from build123d import *

# Parameters (mm, degrees)
BOSS_EXTRUDE1_DEPTH = 19
BOSS_EXTRUDE2_DEPTH = 1
BOSS_EXTRUDE3_DEPTH = 1
SKETCH4_W           = 11
SKETCH4_H           = 15.2
SKETCH4_W_2         = 9
SKETCH4_H_2         = 13.2
BOSS_EXTRUDE4_DEPTH = 5
SKETCH5_W           = 9
SKETCH5_H           = 13.2
CUT_EXTRUDE1_DEPTH  = 13


with BuildPart() as part:
    # Sketch1 → Boss-Extrude1 (new body)
    with BuildSketch(Plane(origin=(0, 0, 0), x_dir=(1, 0, 0), z_dir=(0, 1, 0))):
        with BuildLine():
            Line((-13.001443325, 4.911000499), (-13.001443325, -7.088999501))
            Line((-13.001443325, -7.088999501), (-3.408667462, -11.966682937))
            Line((-3.408667462, -11.966682937), (-5.189854063, -11.966682937))
            Line((-5.189854063, -11.966682937), (-14.067067881, -7.452844668))
            Line((-14.067067881, -7.452844668), (-14.067067881, 3.911000499))
            Line((-14.067067881, 3.911000499), (-28.001443325, 3.911000499))
            Line((-28.001443325, 3.911000499), (-28.001443325, -7.452844668))
            ThreePointArc((-28.001443325, -7.452844668), (-26.679370706, -10.644610317), (-23.487605056, -11.966682937))
            Line((-23.487605056, -11.966682937), (-11.742872705, -11.966682937))
            Line((-11.742872705, -11.966682937), (-11.742872705, -12.966682937))
            Line((-11.742872705, -12.966682937), (-23.494591297, -12.966682937))
            ThreePointArc((-23.494591297, -12.966682937), (-27.388523709, -11.353763321), (-29.001443325, -7.459830909))
            Line((-29.001443325, -7.459830909), (-29.001443325, 4.911000499))
            Line((-29.001443325, 4.911000499), (-13.001443325, 4.911000499))
        make_face()
    extrude(amount=BOSS_EXTRUDE1_DEPTH)

    # Sketch2 → Boss-Extrude2 (add)
    with BuildSketch(Plane(origin=(0, 19, 0), x_dir=(1, 0, 0), z_dir=(0, 1, 0))):
        with BuildLine():
            Line((-29.001443325, 4.911000499), (-13.001443325, 4.911000499))
            Line((-13.001443325, 4.911000499), (-13.001443325, -7.088999501))
            Line((-13.001443325, -7.088999501), (-3.408667462, -11.966682937))
            Line((-3.408667462, -11.966682937), (-5.189854063, -11.966682937))
            Line((-5.189854063, -11.966682937), (-11.742872705, -12.966682937))
            Line((-11.742872705, -12.966682937), (-23.494591297, -12.966682937))
            ThreePointArc((-23.494591297, -12.966682937), (-27.388523709, -11.353763321), (-29.001443325, -7.459830909))
            Line((-29.001443325, -7.459830909), (-29.001443325, 4.911000499))
        make_face()
    extrude(amount=-BOSS_EXTRUDE2_DEPTH)

    # Sketch3 → Boss-Extrude3 (add)
    with BuildSketch(Plane(origin=(0, 0, 0), x_dir=(-1, 0, 0), z_dir=(0, -1, 0))):
        with BuildLine():
            Line((29.001443325, -7.459830909), (29.001443325, 4.911000499))
            Line((29.001443325, 4.911000499), (13.001443325, 4.911000499))
            Line((13.001443325, 4.911000499), (13.001443325, -7.088999501))
            Line((13.001443325, -7.088999501), (3.408667462, -11.966682937))
            Line((3.408667462, -11.966682937), (5.189854063, -11.966682937))
            Line((5.189854063, -11.966682937), (14.067067881, -7.452844668))
            Line((14.067067881, -7.452844668), (14.067067881, 3.911000499))
            Line((14.067067881, 3.911000499), (28.001443325, 3.911000499))
            Line((28.001443325, 3.911000499), (28.001443325, -7.452844668))
            ThreePointArc((28.001443325, -7.452844668), (26.679370706, -10.644610317), (23.487605056, -11.966682937))
            Line((23.487605056, -11.966682937), (11.742872705, -11.966682937))
            Line((11.742872705, -11.966682937), (11.742872705, -12.966682937))
            Line((11.742872705, -12.966682937), (23.494591297, -12.966682937))
            ThreePointArc((23.494591297, -12.966682937), (27.388523709, -11.353763321), (29.001443325, -7.459830909))
        make_face()
        with BuildLine():
            Line((11.742872705, -12.966682937), (3.408667462, -11.966682937))
            Line((3.408667462, -11.966682937), (5.189854063, -11.966682937))
            Line((5.189854063, -11.966682937), (14.067067881, -7.452844668))
            Line((14.067067881, -7.452844668), (14.067067881, 3.911000499))
            Line((14.067067881, 3.911000499), (28.001443325, 3.911000499))
            Line((28.001443325, 3.911000499), (28.001443325, -7.452844668))
            ThreePointArc((28.001443325, -7.452844668), (26.679370706, -10.644610317), (23.487605056, -11.966682937))
            Line((23.487605056, -11.966682937), (11.742872705, -11.966682937))
            Line((11.742872705, -11.966682937), (11.742872705, -12.966682937))
        make_face()
    extrude(amount=-BOSS_EXTRUDE3_DEPTH)

    # Sketch4 → Boss-Extrude4 (add)
    with BuildSketch(Plane(origin=(0, 0, -4.911000499), x_dir=(-1, 0, 0), z_dir=(0, 0, -1))):
        with Locations((21.001443325, 9.5)):
            Rectangle(SKETCH4_W, SKETCH4_H)
        with Locations((21.001443325, 9.5)):
            Rectangle(SKETCH4_W_2, SKETCH4_H_2, mode=Mode.SUBTRACT)
    extrude(amount=BOSS_EXTRUDE4_DEPTH)

    # Sketch5 → Cut-Extrude1 (cut)
    with BuildSketch(Plane(origin=(0, 0, -9.911000499), x_dir=(-1, 0, 0), z_dir=(0, 0, -1))):
        with Locations((21.001443325, 9.5)):
            Rectangle(SKETCH5_W, SKETCH5_H)
    extrude(amount=-CUT_EXTRUDE1_DEPTH, mode=Mode.SUBTRACT)


solid = part.part
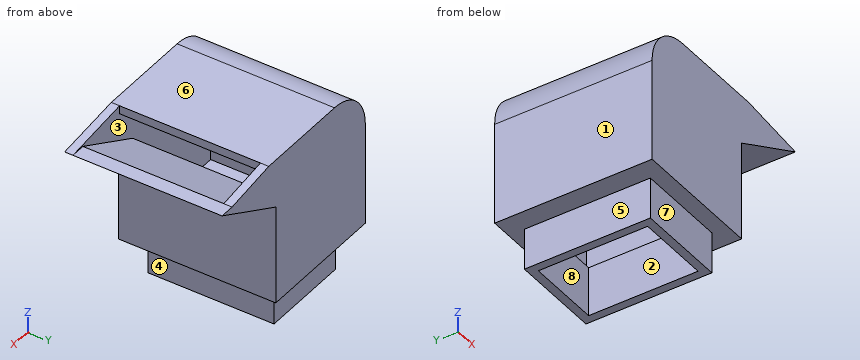
Verification items for the finished model (mm, model axes). Face numbers are marked on the shaded views. A direction names the side the tool comes from. Give positions to 0.01 mm unless a question says otherwise; leave off trailing zeros. Order: outer loops, then holes, each group sorted by start corner. A loop starts at its lowest first (then second) coordinate and runs counter-clockwise, first axis right, second up. Notation, with made-up numbers: M -24,35.5 L 28,35.5 A20 cw 28,44.5 Z; hole C 6.5,-7 d8. An arc over 180 degrees is marked long. Answer as a JSON object with one key per item and string values. Group by question number.
1) Scan lines: line 1 along X through (y, z) = (15.5, 2.75); line 2 along Y through (x, z) = (-23, 4.5); line 3 along X through (y, z) = (15.75, -4). Record each from-to range of solid material in increasing order. Write a range as [from, to].
2) Access from +Z, -Z, +X, -X, +Y, -Y to the whole of each face (thin tool, end or side, straight path). Record for the marked faces 1, 2, 3, 4 and 5.
3) Depth check by flat-ended pin: pin 1 Ø5.5 at (y, z) = (9, 0.5) entering from +X; pin 2 Ø0.8 at (y, z) = (10, 12.5) entering from +X; pin 3 Ø0.5 at (x, y) = (-4, 11) entering from +Z. Enter the tip coordinate at first touch or a pass-through.
4) Mould release check, pull along Y, two halves, no side actions. Record for the marked faces 6, 7 and 8: released by +Y, released by -Y, zero draft, split by the parting line, or undercut.
5) Cross-section at B-B (y = 11.75). Enter the section's corners in (x, z).
6) Cross-section at C-C (x = -19.5). Enter the section's corners in (y, z), then the cut area to 3 significant figures.
7) Cross-section at D-D (z = -0.25). Enter the section's corners in (x, y).
8) Cross-section at A-A (z = -5.75). Enter the section's corners in (x, y), then the cut area to 3 significant figures.
Result sheet:
{
 "1": {"line 1": "x = [-29, -28], [-14.07, -13]", "line 2": "y = [0, 1], [18, 19]", "line 3": "x = [-29, -25.5], [-16.5, -13]"},
 "2": {"face 1": "+Z, -Z, -X, +Y, -Y", "face 2": "-Z", "face 3": "none", "face 4": "-Z, +X, +Y, -Y", "face 5": "-Z, -X, +Y, -Y"},
 "3": {"pin 1": "stops at x = -13", "pin 2": "stops at x = -11.74", "pin 3": "stops at z = 11.97"},
 "4": {"face 6": "zero draft", "face 7": "released by -Y", "face 8": "undercut"},
 "5": {"outline": "M -29,-4.91 L -26.5,-4.91 L -26.5,-9.91 L -25.5,-9.91 L -25.5,-3.91 L -28,-3.91 L -28,7.45 A4.51 cw -23.49,11.97 L -11.74,11.97 L -11.74,12.97 L -23.49,12.97 A5.51 ccw -29,7.46 Z; M -16.5,-9.91 L -15.5,-9.91 L -15.5,-4.91 L -13,-4.91 L -13,7.09 L -3.41,11.97 L -5.19,11.97 L -14.07,7.45 L -14.07,-3.91 L -16.5,-3.91 Z"},
 "6": {"outline": "M 0,-4.91 L 1.9,-4.91 L 1.9,-9.91 L 2.9,-9.91 L 2.9,-3.91 L 1,-3.91 L 1,11.97 L 18,11.97 L 18,-3.91 L 16.1,-3.91 L 16.1,-9.91 L 17.1,-9.91 L 17.1,-4.91 L 19,-4.91 L 19,12.97 L 0,12.97 Z", "area": "66.6 mm2"},
 "7": {"outline": "M -29,0 L -13,0 L -13,19 L -29,19 Z; hole M -28,1 L -14.07,1 L -14.07,18 L -28,18 Z"},
 "8": {"outline": "M -26.5,1.9 L -15.5,1.9 L -15.5,17.1 L -26.5,17.1 Z; hole M -25.5,2.9 L -16.5,2.9 L -16.5,16.1 L -25.5,16.1 Z", "area": "48.4 mm2"}
}
